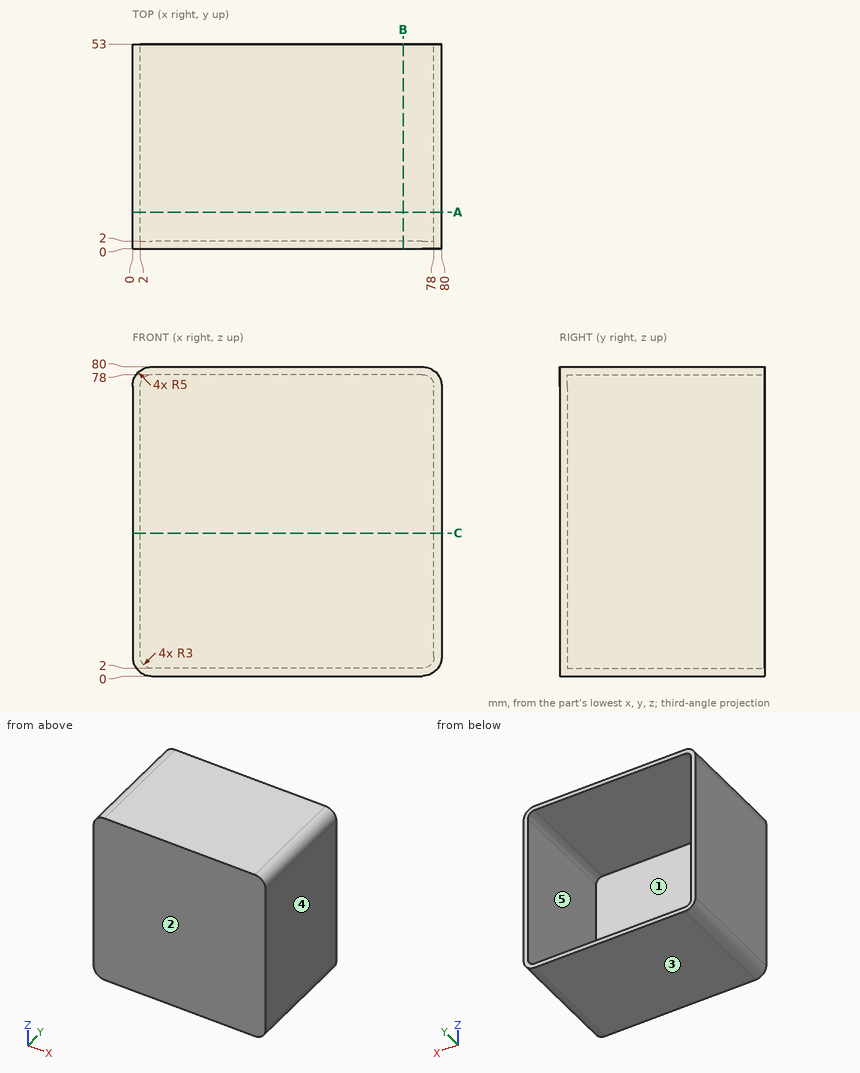
The figure shows three views and two pictorial views of one solid part (mm, origin at its lowest corner). Answer the questions. A direction names the side the tool comes from. Give positions to 0.01 mm unless a question says otherwise; leave off trailing zeros. Write each loop counter-clockwise with the first axis right and the second up, starting at its lowest first coordinate (ties: lowest second). Pieces come first, ordered by that corner, then holes. Notation, with made-up numbers: (48, -28) - (96, -28) arc R25 cw to (96, 11) - close; hole circle Ø3 at (25, -3). An arc over 180 degrees is marked (long way). Use CSV: the item, a comma, the result in double quotes. Start each with the question number.
Item 1: The part is cut by section B-B, the plane x = 70. Give the vertices of the cut face in (y, z), and give its area (3 significant figures).
Item 2: The part is cut by section A-A, the plane y = 9.5. Give the vertices of the cut face in (x, z).
Item 3: For the marked faces 1 and 2, determine the directions among +Z, -Z, +X, -X, +Y, -Y from which every point of the face is accessible in a straight line to the end or side of a thin tool.
Item 4: A flat-ended cylindrical pin translates along its axis: P1, Ø1.5, axis at x = 63, z = 24, coming from the +Y side. Find the tip coordinate at first contact, or state that the pin passes through.
Item 5: The part is cut by section C-C, the plane z = 37. Give the vertices of the cut face in (x, y).
Item 6: Consider line 1 (X direction, y = 29, z = 21); line 2 (Y direction, x = 29, z = 39). Determine where each line is inside the solid, lowest interval first.
Item 7: The mould has two halves that part along X. Classify the marked faces 3, 4 and 5: pulls with the +X half, pulls with the -X half, needs draft (parallel to the pull), parting line crosses it, or undercut.
Taken from the geometry:
1,outline,"(0, 0) - (53, 0) - (53, 2) - (2, 2) - (2, 78) - (53, 78) - (53, 80) - (0, 80) - close"
1,area,"364 mm2"
2,outline,"(0, 5) arc R5 ccw to (5, 0) - (75, 0) arc R5 ccw to (80, 5) - (80, 75) arc R5 ccw to (75, 80) - (5, 80) arc R5 ccw to (0, 75) - close; hole (2, 5) arc R3 ccw to (5, 2) - (75, 2) arc R3 ccw to (78, 5) - (78, 75) arc R3 ccw to (75, 78) - (5, 78) arc R3 ccw to (2, 75) - close"
3,face 1,"+Y"
3,face 2,"+Z, -Z, +X, -X, -Y"
4,P1,"y = 2"
5,outline,"(0, 0) - (80, 0) - (80, 53) - (78, 53) - (78, 2) - (2, 2) - (2, 53) - (0, 53) - close"
6,line 1,"0 to 2, 78 to 80"
6,line 2,"0 to 2"
7,face 3,"needs draft"
7,face 4,"pulls with the +X half"
7,face 5,"undercut"
